Source: CAD feature listing. Evaluate the final solid. Frame: model axes, mm. A direction names the side the tool comes from. Give positions to 0.01 mm unless a question says otherwise; leave off trailing zeros. Order: outer loops, then holes, each group sorted by start corner. A loop starts at its lowest first (then second) coordinate and runs counter-clockwise, first axis right, second up. Notation, with made-up numbers: (32.25, 89) -> (69.25, 89) arc R31 ccw to (69.25, 125) -> close; hole circle Ø10 at (68.25, 4). An arc over 180 degrees is marked (long way). Answer in a Markdown table with one row per item.
```python
from build123d import *

# Parameters (mm, degrees)
SKETCH_1_W          = 58
SKETCH_1_H          = 25
EXTRUDE_1_DEPTH     = 6
SKETCH_2_R          = 4
SKETCH_2_R_2        = 1.65
CUT_EXTRUDE_1_DEPTH = 2
EXTRUDE_2_DEPTH     = 2
SKETCH_4_R          = 1.65
CUT_EXTRUDE_2_DEPTH = 2
EXTRUDE_3_DEPTH     = 4
SKETCH_5_R          = 1.65
EXTRUDE_4_DEPTH     = 4
SKETCH_4_2_R        = 1.65
CUT_EXTRUDE_3_DEPTH = 6
SKETCH_2_2_R        = 4
SKETCH_2_2_R_2      = 1.65
CUT_EXTRUDE_4_DEPTH = 6
CUT_EXTRUDE_5_REACH = 95.421
SKETCH_6_R          = 6
SKETCH_9_W          = 25
SKETCH_9_H          = 40
EXTRUDE_6_DEPTH     = 12.5
SKETCH_10_W         = 25
SKETCH_10_H         = 28
CUT_EXTRUDE_6_DEPTH = 10
FILLET_1_R          = 3


with BuildPart() as part:
    # 草图1 → 凸台-拉伸1 (new body)
    with BuildSketch(Plane(origin=(0, 0, 0), x_dir=(1, 0, 0), z_dir=(0, 1, 0))):
        Rectangle(SKETCH_1_W, SKETCH_1_H)
    extrude(amount=EXTRUDE_1_DEPTH)

    # 草图2 → 切除-拉伸1 (cut)
    with BuildSketch(Plane(origin=(0, 6, 0), x_dir=(1, 0, 0), z_dir=(0, 1, 0))):
        with Locations(Location((0, 0, 0), (0, 0, 270))):
            Circle(SKETCH_2_R)
        with Locations(Location((0, 7, 0), (0, 0, 270))):
            Circle(SKETCH_2_R_2)
        with Locations(Location((7, 0, 0), (0, 0, 270))):
            Circle(SKETCH_2_R_2)
        with Locations(Location((0, -7, 0), (0, 0, 270))):
            Circle(SKETCH_2_R_2)
        with Locations(Location((-7, 0, 0), (0, 0, 270))):
            Circle(SKETCH_2_R_2)
    extrude(amount=-CUT_EXTRUDE_1_DEPTH, mode=Mode.SUBTRACT)

    # 草图3 → 凸台-拉伸2 (add)
    with BuildSketch(Plane(origin=(29, 0, 0), x_dir=(0, 0, -1), z_dir=(1, 0, 0))):
        with BuildLine():
            Line((0, 6), (12.5, 6))
            Line((12.5, 6), (12.5, 80))
            ThreePointArc((12.5, 80), (0, 92.5), (-12.5, 80))
            Line((-12.5, 80), (-12.5, 6))
            Line((-12.5, 6), (0, 6))
        make_face()
    extrude_2 = extrude(amount=-EXTRUDE_2_DEPTH)

    # 草图4 → 切除-拉伸2 (cut)
    with BuildSketch(Plane(origin=(29, 0, 0), x_dir=(0, 0, -1), z_dir=(1, 0, 0))):
        with Locations((0, 87)):
            Circle(SKETCH_4_R)
        with Locations((7, 80)):
            Circle(SKETCH_4_R)
        with Locations((0, 73)):
            Circle(SKETCH_4_R)
        with Locations((-7, 80)):
            Circle(SKETCH_4_R)
        with Locations((0, 80)):
            Circle(SKETCH_4_R)
    cut_extrude_2 = extrude(amount=-CUT_EXTRUDE_2_DEPTH, mode=Mode.SUBTRACT)

    # 镜向1: 凸台-拉伸2, 切除-拉伸2 across plane
    add(extrude_2.mirror(Plane(origin=(0, 0, 0), x_dir=(0, 0, 1), z_dir=(1, 0, 0))))
    add(cut_extrude_2.mirror(Plane(origin=(0, 0, 0), x_dir=(0, 0, 1), z_dir=(1, 0, 0))), mode=Mode.SUBTRACT)

    # 草图3<3> → 凸台-拉伸3 (add)
    with BuildSketch(Plane(origin=(29, 0, 0), x_dir=(0, 0, -1), z_dir=(1, 0, 0))):
        with BuildLine():
            Line((0, 0), (12.5, 0))
            Line((12.5, 0), (12.5, 80))
            ThreePointArc((12.5, 80), (0, 92.5), (-12.5, 80))
            Line((-12.5, 80), (-12.5, 0))
            Line((-12.5, 0), (0, 0))
        make_face()
    extrude(amount=EXTRUDE_3_DEPTH)

    # 草图5 → 凸台-拉伸4 (add)
    with BuildSketch(Plane.ZY.offset(29)):
        with BuildLine():
            Line((-12.5, 0), (12.5, 0))
            Line((12.5, 0), (12.5, 80))
            ThreePointArc((12.5, 80), (0, 92.5), (-12.5, 80))
            Line((-12.5, 80), (-12.5, 0))
        make_face()
        with Locations(Location((0, 73, 0), (0, 0, 180))):
            Circle(SKETCH_5_R, mode=Mode.SUBTRACT)
        with Locations(Location((0, 87, 0), (0, 0, 180))):
            Circle(SKETCH_5_R, mode=Mode.SUBTRACT)
        with Locations(Location((-7, 80, 0), (0, 0, 180))):
            Circle(SKETCH_5_R, mode=Mode.SUBTRACT)
        with Locations(Location((0, 80, 0), (0, 0, 180))):
            Circle(SKETCH_5_R, mode=Mode.SUBTRACT)
        with Locations(Location((7, 80, 0), (0, 0, 180))):
            Circle(SKETCH_5_R, mode=Mode.SUBTRACT)
    extrude(amount=EXTRUDE_4_DEPTH)

    # 草图4<2> → 切除-拉伸3 (cut)
    with BuildSketch(Plane(origin=(29, 0, 0), x_dir=(0, 0, -1), z_dir=(1, 0, 0))):
        with Locations((0, 87)):
            Circle(SKETCH_4_2_R)
        with Locations((7, 80)):
            Circle(SKETCH_4_2_R)
        with Locations((0, 73)):
            Circle(SKETCH_4_2_R)
        with Locations((-7, 80)):
            Circle(SKETCH_4_2_R)
        with Locations((0, 80)):
            Circle(SKETCH_4_2_R)
    extrude(amount=CUT_EXTRUDE_3_DEPTH, mode=Mode.SUBTRACT)

    # 草图2<2> → 切除-拉伸4 (cut)
    with BuildSketch(Plane(origin=(0, 6, 0), x_dir=(1, 0, 0), z_dir=(0, 1, 0))):
        with Locations(Location((0, 0, 0), (0, 0, 270))):
            Circle(SKETCH_2_2_R)
        with Locations(Location((0, 7, 0), (0, 0, 270))):
            Circle(SKETCH_2_2_R_2)
        with Locations(Location((7, 0, 0), (0, 0, 270))):
            Circle(SKETCH_2_2_R_2)
        with Locations(Location((0, -7, 0), (0, 0, 270))):
            Circle(SKETCH_2_2_R_2)
        with Locations(Location((-7, 0, 0), (0, 0, 270))):
            Circle(SKETCH_2_2_R_2)
    extrude(amount=-CUT_EXTRUDE_4_DEPTH, mode=Mode.SUBTRACT)

    # 草图6 → 切除-拉伸5 (cut, up to next)
    with BuildSketch(Plane(origin=(0, 6, 0), x_dir=(1, 0, 0), z_dir=(0, 1, 0)), mode=Mode.PRIVATE) as cut_extrude_5_sk1:
        with Locations(Location((-18, 0, 0), (0, 0, 270))):
            Circle(SKETCH_6_R)
    cut_extrude_5_tool1 = extrude(cut_extrude_5_sk1.sketch, amount=-CUT_EXTRUDE_5_REACH, mode=Mode.PRIVATE) & part.part
    # 草图6 → 切除-拉伸5 (cut, up to next)
    with BuildSketch(Plane(origin=(0, 6, 0), x_dir=(1, 0, 0), z_dir=(0, 1, 0)), mode=Mode.PRIVATE) as cut_extrude_5_sk2:
        with Locations(Location((18, 0, 0), (0, 0, 270))):
            Circle(SKETCH_6_R)
    cut_extrude_5_tool2 = extrude(cut_extrude_5_sk2.sketch, amount=-CUT_EXTRUDE_5_REACH, mode=Mode.PRIVATE) & part.part
    add(cut_extrude_5_tool1.solids().sort_by_distance((-18, 6, 0))[0], mode=Mode.SUBTRACT)
    add(cut_extrude_5_tool2.solids().sort_by_distance((18, 6, 0))[0], mode=Mode.SUBTRACT)

    # 草图9 → 凸台-拉伸6 (add)
    with BuildSketch(Plane(origin=(33, 0, 0), x_dir=(0, 0, -1), z_dir=(1, 0, 0))):
        with Locations((0, 20)):
            Rectangle(SKETCH_9_W, SKETCH_9_H)
    extrude_6 = extrude(amount=EXTRUDE_6_DEPTH)

    # 镜向2: 凸台-拉伸6 across plane
    add(extrude_6.mirror(Plane(origin=(0, 0, 0), x_dir=(0, 0, 1), z_dir=(1, 0, 0))))

    # 草图10 → 切除-拉伸6 (cut)
    with BuildSketch(Plane.ZY.offset(-27)):
        with Locations((0, 20)):
            Rectangle(SKETCH_10_W, SKETCH_10_H)
    cut_extrude_6 = extrude(amount=-CUT_EXTRUDE_6_DEPTH, mode=Mode.SUBTRACT)

    # 镜向3: 切除-拉伸6 across plane
    add(cut_extrude_6.mirror(Plane(origin=(0, 0, 0), x_dir=(0, 0, 1), z_dir=(1, 0, 0))), mode=Mode.SUBTRACT)

    # 圆角1
    fillet_1_edges = [part.edges().sort_by_distance(p)[0] for p in [
        (45.5, 40, 0),
        (-45.5, 40, 0),
        (27, 34, 0),
        (-27, 34, 0),
    ]]
    fillet(fillet_1_edges, radius=FILLET_1_R)


solid = part.part
```
(1) Pull-direction query (Z, two-part tool) for faces 1 (the cylindrical face through (-29.958, 92.497, 0.275)), 2 (the flat face through (33, 67, 0)), 3 (the cylindrical face through (30, 78.4, -6.6)), 4 (the cylindrical face through (5.4, 3, -0.4)); classes: +Z half, -Z half, draft (parallel to the pull), parting line (faces both ways), or undercut.
A:
| item | result |
|---|---|
| face 1 | parting line |
| face 2 | draft |
| face 3 | undercut |
| face 4 | undercut |
(2) First-contact query: pin 1 Ø4.5 at (y, z) = (87, 0) entering from -X; pin 2 Ø5.5 at (x, z) = (-7, 0) entering from +Y; pin 3 Ø4 at (y, z) = (73, 0) entering from +X. Flat tips, straight axial feed; report the tip coordinate or a pass-through.
A:
| item | result |
|---|---|
| pin 1 | stops at x = -33 |
| pin 2 | stops at y = 6 |
| pin 3 | stops at x = 33 |
(3) Section query C-C (y = 20). Return the cut outline in (x, z), plus the area to 3 significant figures.
A:
| item | result |
|---|---|
| outline | (-45.5, -12.5) -> (-37, -12.5) -> (-37, 12.5) -> (-45.5, 12.5) -> close; (37, -12.5) -> (45.5, -12.5) -> (45.5, 12.5) -> (37, 12.5) -> close |
| area | 425 mm^2 |
(4) Access query for faces 5 (the flat face through (37, 20, 0)), 6 (the flat face through (-33, 67, 0)), 7 (the cylindrical face through (30, 78.4, 7.4)), 8 (the flat face through (27, 65, 0)). Directions: +Z, -Z, +X, -X, +Y, -Y. A direction counts if a zero-diameter tool reaches every point of the face in a straight line with its end or side. Return the directions, or none.
A:
| item | result |
|---|---|
| face 5 | +Z, -Z |
| face 6 | +Z, -Z, -X, +Y |
| face 7 | +X, -X |
| face 8 | +Z, -Z, +Y |
(5) Section query B-B (y = 73). Return the cut outline in (x, z).
A:
| item | result |
|---|---|
| outline | (-33, -12.5) -> (-27, -12.5) -> (-27, -1.65) -> (-33, -1.65) -> close; (-33, 1.65) -> (-27, 1.65) -> (-27, 12.5) -> (-33, 12.5) -> close; (27, -12.5) -> (33, -12.5) -> (33, -1.65) -> (27, -1.65) -> close; (27, 1.65) -> (33, 1.65) -> (33, 12.5) -> (27, 12.5) -> close |
(6) Ray query, probe 1 along Z at (x, y) = (-29, 80); probe 2 along X at (y, z) = (1.75, 0); probe 3 along Y at (x, z) = (-30.4, 0). Return the intervals inside material, ascending.
A:
| item | result |
|---|---|
| probe 1 | z = -12.5 to -8.65, -5.35 to -1.65, 1.65 to 5.35, 8.65 to 12.5 |
| probe 2 | x = -45.5 to -24, -12 to -8.65, -5.35 to -4, 4 to 5.35, 8.65 to 12, 24 to 45.5 |
| probe 3 | y = 0 to 6, 34 to 71.35, 74.65 to 78.35, 81.65 to 85.35, 88.65 to 92.5 |
(7) Section query D-D (z = 0). Give the number of separate pieces and of enclosed holes in the cut face, plus the area to 3 significant figures.
A:
| item | result |
|---|---|
| separate pieces | 12 |
| enclosed holes | 0 |
| area | 1,520 mm^2 |
(8) Section query A-A (x = 7). Return the cut outline in (y, z), plus the area to 3 significant figures.
A:
| item | result |
|---|---|
| outline | (0, -12.5) -> (6, -12.5) -> (6, -1.65) -> (0, -1.65) -> close; (0, 1.65) -> (6, 1.65) -> (6, 12.5) -> (0, 12.5) -> close |
| area | 130 mm^2 |
